Study the drawing (mm; zero at the part's minimum x, y, z) and answer. Coordinates: 2 decimals unless noted, no trailing zeros. Loops run counter-clockwise (first coordinate to the right, second up) from the corner with the lowest first, then second, coordinate; pieces in that order, holes last. Notation, with made-up numbers: (4.5, -30.5) - (26.5, -30.5) arc R31 ccw to (26.5, 1.5) - close; hole circle Ø2 at (82.5, -16.75). An arc over 180 degrees is marked (long way). Use one line per item in the form item = value.
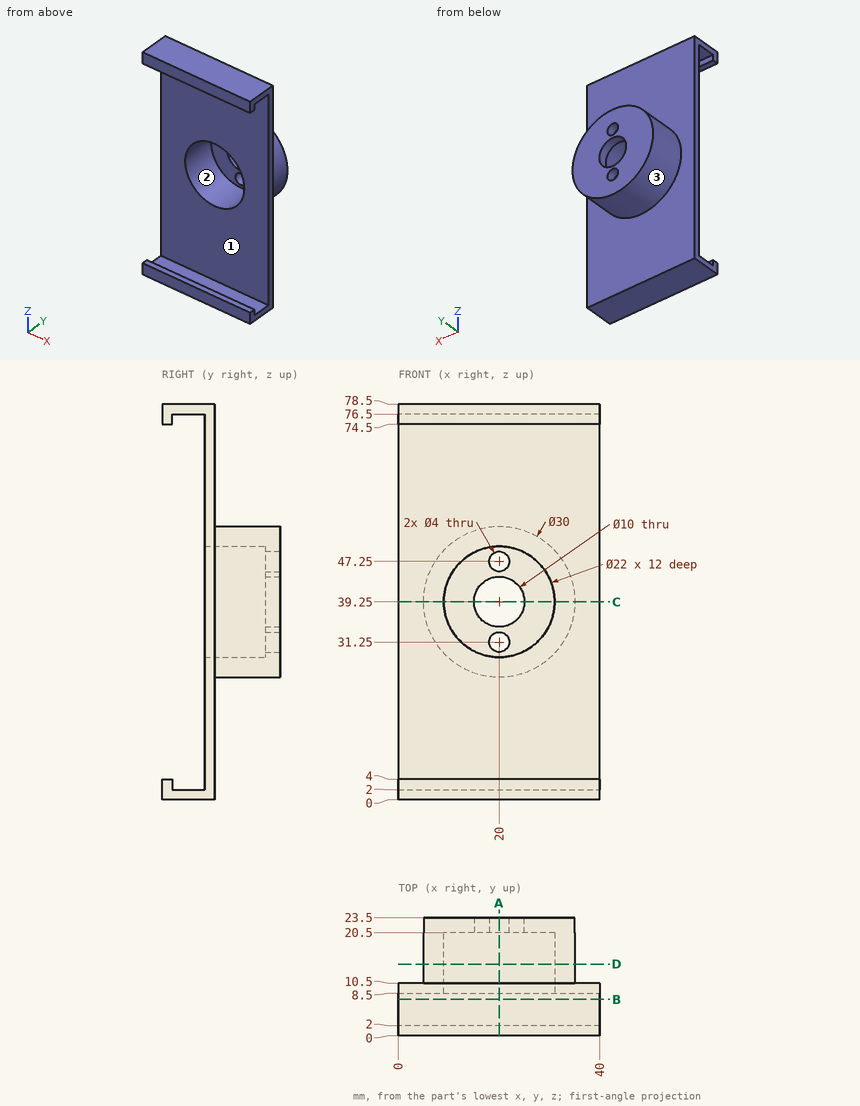
Item 1: The part is cut by section B-B on y = 7.25. Give the vertices of the cut face in (x, z), plus the area to 3 significant figures.
Results below:
outline = (0, 0) - (40, 0) - (40, 2) - (0, 2) - close; (0, 76.5) - (40, 76.5) - (40, 78.5) - (0, 78.5) - close
area = 160 mm²
Item 2: For a pull along X with two mould halves and no side action, classify the marked faces 1, 2 and 3 as +X half, -X half, draft (parallel to the pull), parting line (faces both ways), or undercut.
Results below:
face_1 = draft
face_2 = undercut
face_3 = parting line
Item 3: Find the intervals of material crossed by L1, parallel to Z at x = 20, y = 22.2; L2, parallel to Z at x = 20, y = 11.25; L3, parallel to X at y = 14.75, z = 39.25, in increasing order.
Results below:
L1 = 24.25 to 29.25, 33.25 to 34.25, 44.25 to 45.25, 49.25 to 54.25
L2 = 24.25 to 28.25, 50.25 to 54.25
L3 = 5 to 9, 31 to 35
Item 4: The part is cut by section D-D on y = 14.25. Give the vertices of the cut face in (x, z), plus the area to 3 significant figures.
Results below:
outline = circle Ø30 at (20, 39.25); hole circle Ø22 at (20, 39.25)
area = 327 mm²
Item 5: The part is cut by section A-A on x = 20. Count the separate pieces of the cut face and the enclosed holes in it, plus the area to 3 significant figures.
Results below:
separate_pieces = 4
enclosed_holes = 0
area = 271 mm²
Item 6: Each of these flat-tipped pins is pushed along its axis until it touches: P1, Ø7, axis at x = 25, y = 6.5, coming from the -Z side; P2, Ø4, axis at x = 28, z = 13.5, coming from the -Y side; P3, Ø2, axis at x = 28, z = 76, coming from the +Y side; P4, Ø13, axis at x = 20, z = 39.25, coming from the -Y side. Where does it stop, or does it pass through?
Results below:
P1 = 0
P2 = 8.5
P3 = 10.5
P4 = 20.5
Item 7: The part is cut by section C-C on z = 39.25. Give the vertices of the cut face in (x, y).
Results below:
outline = (0, 8.5) - (9, 8.5) - (9, 20.5) - (15, 20.5) - (15, 23.5) - (5, 23.5) - (5, 10.5) - (0, 10.5) - close; (25, 20.5) - (31, 20.5) - (31, 8.5) - (40, 8.5) - (40, 10.5) - (35, 10.5) - (35, 23.5) - (25, 23.5) - close
